from build123d import *

# Parameters (mm, degrees)
SKETCH1_W           = 110
SKETCH1_H           = 80
BOSS_EXTRUDE1_DEPTH = 2
SKETCH2_R           = 1.624633008
CUT_EXTRUDE1_DEPTH  = 69.036754773


with BuildPart() as part:
    # Sketch1 → Boss-Extrude1 (new body)
    with BuildSketch(Plane.XY):
        Rectangle(SKETCH1_W, SKETCH1_H)
    extrude(amount=-BOSS_EXTRUDE1_DEPTH)

    # Sketch2 → Cut-Extrude1 (cut, through all)
    with BuildSketch(Plane.XY):
        with Locations((-50, 34)):
            Circle(SKETCH2_R)
        with Locations(Location((50, 34, 0), (0, 0, 180))):
            Circle(SKETCH2_R)
        with Locations((50, -34)):
            Circle(SKETCH2_R)
        with Locations(Location((-50, -34, 0), (0, 0, 180))):
            Circle(SKETCH2_R)
    extrude(amount=-CUT_EXTRUDE1_DEPTH, mode=Mode.SUBTRACT)


solid = part.part
Source: CAD feature listing. Evaluate the final solid. Frame: model axes, mm. Round coordinates to 2 decimals unless told otherwise and drop trailing zeros. Loops run counter-clockwise (first coordinate to the right, second up) from the corner with the lowest first, then second, coordinate; pieces in that order, holes last.
Q1. Section B-B, the plane y = -34. Return loops of the section in (x, z).
Q2. First-contact query: P1, Ø8, axis at x = 1, y = -4, coming from the +Z side; P2, Ø2.5, axis at x = -50, y = 34, coming from the +Z side. Flat tips, straight axial feed; report the tip coordinate or a pass-through.
Q3. Section A-A, the plane x = -50. Return loops of the section in (y, z).
Q4. Ray query, line 1 (Y direction, x = -50, z = -1.05); line 2 (X direction, y = -33, z = -0.75). Return the intervals inside material, ascending.
Q5. Mould query, pull axis X, two halves, no side actions, for faces 1 (the face through (-1, 1, 0)), 2 (the face through (-48.45, 34.49, -0.99)). Classes: pulls with the +X half, pulls with the -X half, needs draft (parallel to the pull), parting line crosses it, or undercut.
Solutions:
1. outline: (-55, -2) - (-51.62, -2) - (-51.62, 0) - (-55, 0) - close; (-48.38, -2) - (48.38, -2) - (48.38, 0) - (-48.38, 0) - close; (51.62, -2) - (55, -2) - (55, 0) - (51.62, 0) - close
2. P1: stops at z = 0
2. P2: passes through
3. outline: (-40, -2) - (-35.62, -2) - (-35.62, 0) - (-40, 0) - close; (-32.38, -2) - (32.38, -2) - (32.38, 0) - (-32.38, 0) - close; (35.62, -2) - (40, -2) - (40, 0) - (35.62, 0) - close
4. line 1: y = -40 to -35.62, -32.38 to 32.38, 35.62 to 40
4. line 2: x = -55 to -51.28, -48.72 to 48.72, 51.28 to 55
5. face 1: needs draft
5. face 2: undercut
